Read the model definition and answer for the solid it produces. Units are mm, in the model's axes. A direction names the side the tool comes from. Round coordinates to 2 decimals unless told otherwise and drop trailing zeros. Order: outer loops, then holes, each group sorted by start corner. A loop starts at its lowest first (then second) coordinate and runs counter-clockwise, first axis right, second up. Notation, with made-up numbers: (28, 60.5) -> (52, 60.5) arc R18 ccw to (52, 77.5) -> close; hole circle Ø2 at (81.25, -15). An arc over 180 degrees is marked (long way). One line per item, written item: value. Start each with the question number.
1. A flat-ended cylindrical pin translates along its axis: pin 1 Ø16 at (x, y) = (40, 15) entering from +Z. Find the tip coordinate at first contact, or state that the pin passes through.
2. Consider line 1 (Y direction, x = 40, z = 5.75); line 2 (X direction, y = -2.5, z = 9); line 3 (X direction, y = -19.5, z = 8). Determine where each line is inside the solid, lowest interval first.
3. Section B-B (x = 43) is taken. Give the vertices of the cut face in (y, z), then the cut area to 3 significant figures.
4. Section D-D (y = 0) is taken. Give the vertices of the cut face in (x, z), then the cut area to 3 significant figures.
5. The mould has two halves that part along Y. Classify faces 1 (the face through (-1, 25, 5)), 2 (the face through (-1, -25, 5)), 3 (the face through (-44.712, 0, 5)): released by +Y, released by -Y, zero draft, split by the parting line, or undercut.
6. Section C-C (z = 7.5) is taken. Give the vertices of the cut face in (x, y), then the cut area to 3 significant figures.
7. For faces 4 (the face through (-50, 0, 5)), 5 (the face through (-41.51, 5.6, 4.93)), determine the directions among +Z, -Z, +X, -X, +Y, -Y from which every point of the face is accessible in a straight line to the end or side of a thin tool.
8. Section A-A (y = 15) is taken. Give the vertices of the cut face in (x, z).
from build123d import *

# Parameters (mm, degrees)
F0_W     = 100
F0_H     = 50
F0_R     = 5
F1_DEPTH = 10


with BuildPart() as f1:
    # F0 (on Top) → F1 (new body)
    with BuildSketch(Plane.XY):
        Rectangle(F0_W, F0_H)
        with Locations((40, -15)):
            Circle(F0_R, mode=Mode.SUBTRACT)
        Polygon((-31.711863, 3.752777), (-31.711863, -3.752777), (-38.211863, -7.505553), (-44.711863, -3.752777), (-44.711863, 3.752777), (-38.211863, 7.505553), align=None, mode=Mode.SUBTRACT)
        with Locations((40, 15)):
            Circle(F0_R, mode=Mode.SUBTRACT)
    extrude(amount=F1_DEPTH)


solid = f1.part
Answer:
1. pin 1: z = 10
2. line 1: -25 to -20, -10 to 10, 20 to 25
2. line 2: -50 to -44.71, -31.71 to 50
2. line 3: -50 to 37.82, 42.18 to 50
3. outline: (-25, 0) -> (-19, 0) -> (-19, 10) -> (-25, 10) -> close; (-11, 0) -> (11, 0) -> (11, 10) -> (-11, 10) -> close; (19, 0) -> (25, 0) -> (25, 10) -> (19, 10) -> close
3. area: 340 mm^2
4. outline: (-50, 0) -> (-44.71, 0) -> (-44.71, 10) -> (-50, 10) -> close; (-31.71, 0) -> (50, 0) -> (50, 10) -> (-31.71, 10) -> close
4. area: 870 mm^2
5. face 1: released by +Y
5. face 2: released by -Y
5. face 3: undercut
6. outline: (-50, -25) -> (50, -25) -> (50, 25) -> (-50, 25) -> close; hole (-44.71, -3.75) -> (-38.21, -7.51) -> (-31.71, -3.75) -> (-31.71, 3.75) -> (-38.21, 7.51) -> (-44.71, 3.75) -> close; hole circle Ø10 at (40, -15); hole circle Ø10 at (40, 15)
6. area: 4,700 mm^2
7. face 4: +Z, -Z, -X, +Y, -Y
7. face 5: +Z, -Z
8. outline: (-50, 0) -> (35, 0) -> (35, 10) -> (-50, 10) -> close; (45, 0) -> (50, 0) -> (50, 10) -> (45, 10) -> close
